Design review of the part built by this model. Coordinates are the model's own, in mm. Give positions to 0.01 mm unless a question says otherwise; leave off trailing zeros. Loops run counter-clockwise (first coordinate to the right, second up) from the corner with the lowest first, then second, coordinate; pieces in that order, holes last. Notation, with made-up numbers: (54.5, 57) -> (58.5, 57) arc R17 ccw to (58.5, 84) -> close; hole circle Ø5 at (45.5, 70.5). An arc over 180 degrees is marked (long way). Use a Markdown table: item, result. Add a question column.
1. Add section C-C (x = -0.75). State the section outline as (y, z) points, and give its area (3 significant figures).
2. Add section B-B (y = 0). State the section outline as (x, z) points.
3. For pin 1 Ø1.5 at (y, z) = (2.5, 6.5) entering from -X, flat-tipped, find the tip position at first contact; note if it passes through.
4. Add section D-D (y = 2.5). State the section outline as (x, z) points, and give its area (3 significant figures).
5. To check wall thickness, follow line 1 (X direction, y = 0, z = 9.9); line 2 (X direction, y = -0.25, z = 4); line 3 (Y direction, x = -0.85, z = 8). State the ranges of each line that lie inside material, in increasing order.
6. Add section A-A (z = 3.75). State the section outline as (x, y) points, and give its area (3 significant figures).
Autodesk Inventor part; units mm, degrees
ref_plane "YZ Plane" through (0, 0, 0) normal (1, 0, 0) x (0, 1, 0)
ref_plane "XZ Plane" through (0, 0, 0) normal (0, 1, 0) x (-1, 0, 0)
ref_plane "XY Plane" through (0, 0, 0) normal (0, 0, 1) x (1, 0, 0)
sketch "スケッチ1" plane through (0, 0, 0) normal (0, 0, 1) x (1, 0, 0)
  line L0 (0, 2.8868) -> (2.5, 1.4434)
  line L1 (2.5, 1.4434) -> (2.5, -1.4434)
  line L2 (2.5, -1.4434) -> (0, -2.8868)
  line L3 (0, -2.8868) -> (-2.5, -1.4434)
  line L4 (-2.5, -1.4434) -> (-2.5, 1.4434)
  line L5 (-2.5, 1.4434) -> (0, 2.8868)
  point P0 (0, 0)
  point P1 (0, 0)
  dimension "d0" = 5
extrude "押し出し1" add sketch "スケッチ1" along normal blind 13.5
sketch "スケッチ2" plane through (0, 0, 13.5) normal (0, 0, 1) x (1, 0, 0)
  point P0 (0, 0)
hole "穴1" at (0, 0, 13.5) direction (0, 0, -1) diameter 2.113 depth 7.6 tip angle 118
sketch "スケッチ3" plane through (0, 0, 0) normal (0, 0, -1) x (-1, 0, 0)
  point P0 (0, 0)
hole "穴2" at (0, 0, 0) direction (0, 0, 1) diameter 2.113 depth 7.6 tip angle 118
properties part number "黄銅スペーサー（六角）_ASB-2613.5E" material "真鍮、ソフト イエロー"
Taken from the geometry:
| question | item | result |
|---|---|---|
| 1 | outline | (-2.45, 0) -> (-0.74, 0) -> (-0.74, 13.5) -> (-2.45, 13.5) -> close; (0.74, 0) -> (2.45, 0) -> (2.45, 13.5) -> (0.74, 13.5) -> close |
| 1 | area | 46.2 mm^2 |
| 2 | outline | (-2.5, 0) -> (-1.06, 0) -> (-1.06, 13.5) -> (-2.5, 13.5) -> close; (1.06, 0) -> (2.5, 0) -> (2.5, 13.5) -> (1.06, 13.5) -> close |
| 3 | pin 1 | stops at x = -1.97 |
| 4 | outline | (-0.67, 0) -> (0.67, 0) -> (0.67, 13.5) -> (-0.67, 13.5) -> close |
| 4 | area | 18.1 mm^2 |
| 5 | line 1 | x = -2.5 to -1.06, 1.06 to 2.5 |
| 5 | line 2 | x = -2.5 to -1.03, 1.03 to 2.5 |
| 5 | line 3 | y = -2.4 to -0.63, 0.63 to 2.4 |
| 6 | outline | (-2.5, -1.44) -> (0, -2.89) -> (2.5, -1.44) -> (2.5, 1.44) -> (0, 2.89) -> (-2.5, 1.44) -> close; hole circle Ø2.11 at (0, 0) |
| 6 | area | 18.1 mm^2 |
